Autodesk Inventor part; units mm, degrees
ref_plane "screw_m25_2_XY" through (0, -13.462, -10.16) normal (0, 1, 0) x (1, 0, 0)
ref_plane "screw_m25_2_YZ" through (0, -13.462, -10.16) normal (1, 0, 0) x (0, 0, -1)
ref_plane "screw_m25_2_ZX" through (0, -13.462, -10.16) normal (0, 0, -1) x (0, 1, 0)
sketch "Sketch_1" plane through (0, 0, 0) normal (0, 1, 0) x (-1, 0, 0)
  line L0 (8.8011, -13.3858) -> (8.8011, 13.3858)
  arc A0 (8.8011, 13.3858) -> (8.2931, 13.8938) centre (8.2931, 13.3858) ccw
  line L1 (8.2931, 13.8938) -> (-8.2931, 13.8938)
  arc A1 (-8.2931, 13.8938) -> (-8.8011, 13.3858) centre (-8.2931, 13.3858) ccw
  line L2 (-8.8011, 13.3858) -> (-8.8011, -13.3858)
  arc A2 (-8.8011, -13.3858) -> (-8.2931, -13.8938) centre (-8.2931, -13.3858) ccw
  line L3 (-8.2931, -13.8938) -> (8.2931, -13.8938)
  arc A3 (8.2931, -13.8938) -> (8.8011, -13.3858) centre (8.2931, -13.3858) ccw
extrude "Extrusion1" add sketch "Sketch_1" against normal blind 15.494
sketch "Sketch_2" plane through (0, -15.494, 0) normal (0, 1, 0) x (1, 0, 0)
  arc A0 (-4.953, -12.446) -> (-4.699, -12.7) centre (-4.699, -12.446) ccw
  line L0 (-4.699, -12.7) -> (-4.318, -12.7)
  line L1 (-4.318, -12.7) -> (-4.318, -8.89)
  line L2 (-4.318, -8.89) -> (-4.699, -8.89)
  arc A1 (-4.699, -8.89) -> (-4.953, -9.144) centre (-4.699, -9.144) ccw
  line L3 (-4.953, -9.144) -> (-4.953, -12.446)
extrude "Extrusion2" cut sketch "Sketch_2" along normal blind 0.254
sketch "Sketch_3" plane through (0, -15.494, 0) normal (0, 1, 0) x (1, 0, 0)
  line L0 (4.318, -12.7) -> (4.699, -12.7)
  arc A0 (4.699, -12.7) -> (4.953, -12.446) centre (4.699, -12.446) ccw
  line L1 (4.953, -12.446) -> (4.953, -9.144)
  arc A1 (4.953, -9.144) -> (4.699, -8.89) centre (4.699, -9.144) ccw
  line L2 (4.699, -8.89) -> (4.318, -8.89)
  line L3 (4.318, -8.89) -> (4.318, -12.7)
extrude "Extrusion3" cut sketch "Sketch_3" along normal blind 0.254
sketch "Sketch_4" plane through (0, -15.494, 0) normal (0, 1, 0) x (1, 0, 0)
  line L0 (-4.953, 12.446) -> (-4.953, 9.144)
  arc A0 (-4.953, 9.144) -> (-4.699, 8.89) centre (-4.699, 9.144) ccw
  line L1 (-4.699, 8.89) -> (-4.318, 8.89)
  line L2 (-4.318, 8.89) -> (-4.318, 12.7)
  line L3 (-4.318, 12.7) -> (-4.699, 12.7)
  arc A1 (-4.699, 12.7) -> (-4.953, 12.446) centre (-4.699, 12.446) ccw
extrude "Extrusion4" cut sketch "Sketch_4" along normal blind 0.254
sketch "Sketch_5" plane through (0, -15.494, 0) normal (0, 1, 0) x (1, 0, 0)
  line L0 (4.318, 12.7) -> (4.318, 8.89)
  line L1 (4.318, 8.89) -> (4.699, 8.89)
  arc A0 (4.699, 8.89) -> (4.953, 9.144) centre (4.699, 9.144) ccw
  line L2 (4.953, 9.144) -> (4.953, 12.446)
  arc A1 (4.953, 12.446) -> (4.699, 12.7) centre (4.699, 12.446) ccw
  line L3 (4.699, 12.7) -> (4.318, 12.7)
extrude "Extrusion5" cut sketch "Sketch_5" along normal blind 0.254
sketch "Sketch6" plane through (0, -15.494, 0) normal (0, -1, 0) x (1, 0, 0)
  point P0 (0, 10.16)
hole "Drilling 1" at (0, -15.494, 10.16) direction (0, 1, 0) diameter 2.5 depth 15.494 counterbore diameter 5.08 counterbore depth 2.032
sketch "Sketch7" plane through (0, -15.494, 0) normal (0, -1, 0) x (1, 0, 0)
  point P0 (0, -10.16)
hole "Drilling 2" at (0, -15.494, -10.16) direction (0, 1, 0) diameter 2.5 depth 15.494 counterbore diameter 5.08 counterbore depth 2.032
ref_plane "screw_m25_2_XY" through (0, -13.462, -10.16) normal (0, 1, 0) x (1, 0, 0)
ref_plane "screw_m25_2_YZ" through (0, -13.462, -10.16) normal (1, 0, 0) x (0, 0, -1)
ref_plane "screw_m25_2_ZX" through (0, -13.462, -10.16) normal (0, 0, -1) x (0, 1, 0)
ref_plane "sscrew_m25_1_XY" through (0, -13.462, 10.16) normal (0, 1, 0) x (1, 0, 0)
ref_plane "sscrew_m25_1_YZ" through (0, -13.462, 10.16) normal (1, 0, 0) x (0, 0, -1)
ref_plane "sscrew_m25_1_ZX" through (0, -13.462, 10.16) normal (0, 0, -1) x (0, 1, 0)
ref_plane "to_dummy_XY" through (0, 0, 0) normal (0, -1, 0) x (1, 0, 0)
ref_plane "to_dummy_YZ" through (0, 0, 0) normal (1, 0, 0) x (0, 0, 1)
ref_plane "to_dummy_ZX" through (0, 0, 0) normal (0, 0, 1) x (0, -1, 0)
ref_plane "to_electric_XY" through (0, -15.24, 0) normal (0, 1, 0) x (1, 0, 0)
ref_plane "to_electric_YZ" through (0, -15.24, 0) normal (1, 0, 0) x (0, 0, -1)
ref_plane "to_electric_ZX" through (0, -15.24, 0) normal (0, 0, -1) x (0, 1, 0)
ref_plane "to_panel_XY" through (0, 0, 0) normal (0, -1, 0) x (1, 0, 0)
ref_plane "to_panel_YZ" through (0, 0, 0) normal (1, 0, 0) x (0, 0, 1)
ref_plane "to_panel_ZX" through (0, 0, 0) normal (0, 0, 1) x (0, -1, 0)
properties part number "S114-body"
Here's how the part is built. I have some questions about the finished solid (model axes, mm). A direction names the side the tool comes from. Coordinates: 2 decimals unless noted, no trailing zeros. Write each loop counter-clockwise with the first axis right and the second up, starting at its lowest first coordinate (ties: lowest second). Pieces come first, ordered by that corner, then holes. Notation, with made-up numbers: (29, 15.5) -> (76, 15.5) arc R32 ccw to (76, 52.5) -> close; hole circle Ø8 at (55, -35.5). An arc over 180 degrees is marked (long way). Use a Markdown table: item, result. Add a question column.
(1) If we section it at B-B, the plane x = 0: Write out the boundary of the cut face in (y, z).
(2) I'm going to push a flat-ended pin straight in: P1, Ø1.5, axis at x = 0, z = -9.5, coming from the -Y side. Where does the tip first touch, or does it pass through?
(3) For faces 4 (the flat face through (1, -13.462, -9)), 5 (the cylindrical face through (-0.05, -6.64, -8.91)), which set-ups out of +Z, -Z, +X, -X, +Y, -Y let a thin tool reach every point of the face, with its end or its side?
(4) If we section it at A-A, the plane z = 10.16: Write out the boundary of the cut face in (x, y), and give its area (3 significant figures).
(5) If we section it at D-D, the plane z = -8.25: Write out the boundary of the cut face in (x, y).
(6) We'd pull the mould along X, two halves only. Please class faces 1 (the cylindrical face through (0.479, -6.637, 9.005)), 2 (the flat face through (0, 0, 0)), 3 (the flat face through (-8.801, -8, 0)): +X half, -X half, draft (parallel to the pull), parting line (faces both ways), or undercut.
(7) Please list where these lines run through material, in increasing order: line 1 (Z direction, x = 0, y = -8.5); line 2 (Z direction, x = 0, y = -14.8); line 3 (X direction, y = -14.3, z = 10.16).
(8) If we section it at C-C, the plane y = -1.75: Write out the boundary of the cut face in (x, z), and give its area (3 significant figures).
Outcome:
| question | item | result |
|---|---|---|
| 1 | outline | (-15.49, -13.89) -> (0, -13.89) -> (0, -11.41) -> (-13.46, -11.41) -> (-13.46, -12.7) -> (-15.49, -12.7) -> close; (-15.49, -7.62) -> (-13.46, -7.62) -> (-13.46, -8.91) -> (0, -8.91) -> (0, 8.91) -> (-13.46, 8.91) -> (-13.46, 7.62) -> (-15.49, 7.62) -> close; (-15.49, 12.7) -> (-13.46, 12.7) -> (-13.46, 11.41) -> (0, 11.41) -> (0, 13.89) -> (-15.49, 13.89) -> close |
| 2 | P1 | stops at y = -13.46 |
| 3 | face 4 | -Y |
| 3 | face 5 | +Y, -Y |
| 4 | outline | (-8.8, -15.49) -> (-4.95, -15.49) -> (-4.95, -15.24) -> (-4.32, -15.24) -> (-4.32, -15.49) -> (-2.54, -15.49) -> (-2.54, -13.46) -> (-1.25, -13.46) -> (-1.25, 0) -> (-8.8, 0) -> close; (1.25, -13.46) -> (2.54, -13.46) -> (2.54, -15.49) -> (4.32, -15.49) -> (4.32, -15.24) -> (4.95, -15.24) -> (4.95, -15.49) -> (8.8, -15.49) -> (8.8, 0) -> (1.25, 0) -> close |
| 4 | area | 228 mm^2 |
| 5 | outline | (-8.8, -15.49) -> (-1.67, -15.49) -> (-1.67, -13.46) -> (1.67, -13.46) -> (1.67, -15.49) -> (8.8, -15.49) -> (8.8, 0) -> (-8.8, 0) -> close |
| 6 | face 1 | undercut |
| 6 | face 2 | draft |
| 6 | face 3 | -X half |
| 7 | line 1 | z = -13.89 to -11.41, -8.91 to 8.91, 11.41 to 13.89 |
| 7 | line 2 | z = -13.89 to -12.7, -7.62 to 7.62, 12.7 to 13.89 |
| 7 | line 3 | x = -8.8 to -2.54, 2.54 to 8.8 |
| 8 | outline | (-8.8, -13.39) arc R0.51 ccw to (-8.29, -13.89) -> (8.29, -13.89) arc R0.51 ccw to (8.8, -13.39) -> (8.8, 13.39) arc R0.51 ccw to (8.29, 13.89) -> (-8.29, 13.89) arc R0.51 ccw to (-8.8, 13.39) -> close; hole circle Ø2.5 at (0, -10.16); hole circle Ø2.5 at (0, 10.16) |
| 8 | area | 479 mm^2 |
